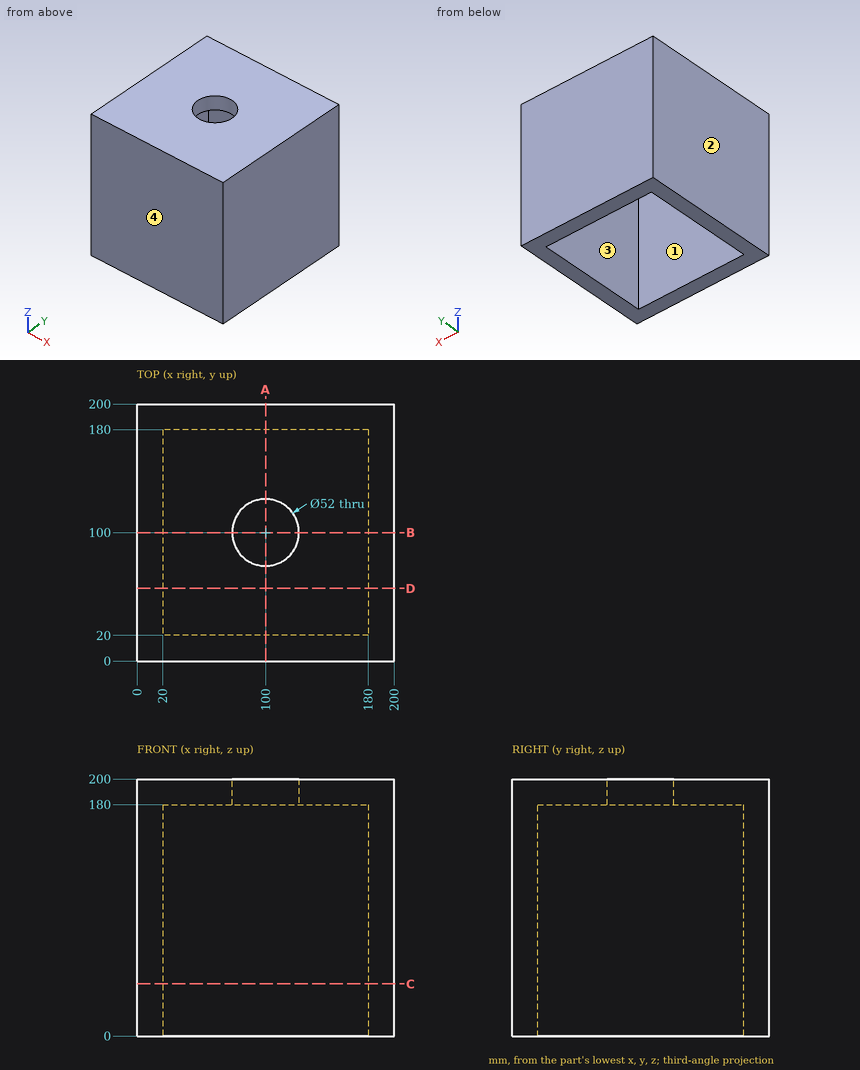
Source: three-view drawing plus pictorial views. Frame: mm from the lowest corner of the part. Round coordinates to 2 decimals unless told otherwise and drop trailing zeros. Order: outer loops, then holes, each group sorted by start corner. A loop starts at its lowest first (then second) coordinate and runs counter-clockwise, first axis right, second up. Notation, with made-up numbers: (-1, 88.25) - (51, 88.25) arc R19 cw to (51, 97.25) - close; hole circle Ø3 at (45, 59). An arc over 180 degrees is marked (long way). Answer in a Markdown table with one row per item.
Item 1: Line query: line 1 (Y direction, x = 100, z = 188.5); line 2 (Y direction, x = 71.5, z = 101). Output: solid intervals per line, ascending.
Model answer:
| item | result |
|---|---|
| line 1 | y = 0 to 74, 126 to 200 |
| line 2 | y = 0 to 20, 180 to 200 |
Item 2: Section query D-D (y = 56.5). Return the cut outline in (x, z).
Model answer:
| item | result |
|---|---|
| outline | (0, 0) - (20, 0) - (20, 180) - (180, 180) - (180, 0) - (200, 0) - (200, 200) - (0, 200) - close |
Item 3: Section query C-C (z = 40.5). Return the cut outline in (x, y), then the cut area to 3 significant figures.
Model answer:
| item | result |
|---|---|
| outline | (0, 0) - (200, 0) - (200, 200) - (0, 200) - close; hole (20, 20) - (180, 20) - (180, 180) - (20, 180) - close |
| area | 14,400 mm² |
Item 4: Mould query, pull axis Y, two halves, no side actions, for the marked faces 1, 2, 3 and 4. Classes: released by +Y, released by -Y, zero draft, split by the parting line, or undercut.
Model answer:
| item | result |
|---|---|
| face 1 | undercut |
| face 2 | zero draft |
| face 3 | undercut |
| face 4 | released by -Y |
Item 5: Section query A-A (x = 100). Return the cut outline in (y, z).
Model answer:
| item | result |
|---|---|
| outline | (0, 0) - (20, 0) - (20, 180) - (74, 180) - (74, 200) - (0, 200) - close; (126, 180) - (180, 180) - (180, 0) - (200, 0) - (200, 200) - (126, 200) - close |
